Input: part model. Units: mm. Frame: model coordinates. A direction names the side the tool comes from. Coordinates: 2 decimals unless noted, no trailing zeros. Write each loop counter-clockwise with the first axis right and the second up, starting at its lowest first coordinate (ties: lowest second). Pieces come first, ordered by that corner, then holes.
1) Section query D-D (x = -4.5). Output: boundary loops of the cut face in (y, z).
2) Section query C-C (z = 0). Output: boundary loops of the cut face in (x, y), then the cut area to 3 significant figures.
3) Section query B-B (y = 0). Output: boundary loops of the cut face in (x, z).
4) Set-up query: faces 4 (the cylindrical face through (-14.32, -0.95, -0.04)), 5 (the flat face through (-14, 1.85, 0)), 6 (the flat face through (-14, -1.85, 0)), 7 (the flat face through (14, -1.85, 0)). Return all of +Z, -Z, +X, -X, +Y, -Y with unobstructed straight access to the full face (end or side cutting, diameter ignored); none if empty.
5) Section query A-A (x = 14). Output: boundary loops of the cut face in (y, z) (3 decimals).
6) Draft query along Z for faces 1 (the cylindrical face through (14.32, -0.95, 0.04)), 2 (the flat face through (14, 1.85, 0)), 3 (the flat face through (10.35, 0, 0)). Return one class per face: pulls with the +Z half, pulls with the -Z half, needs draft (parallel to the pull), parting line crosses it, or undercut.
7) Line query: L1, parallel to Z at x = -13, y = 0; L2, parallel to Y at x = -13.25, z = 0; L3, parallel to Z at x = -4, y = 0.1. Output: solid intervals per line, ascending.
8) Pin query (flat end, axial travel): pin 1 Ø0.8 at (y, z) = (-2.5, -0.5) entering from -X; pin 2 Ø1.8 at (x, z) = (12.5, 0) entering from +Y; pin 3 Ø3 at (x, z) = (14.5, -0.5) entering from -Y. Return the tip coordinate at first contact, or that it passes through.
from build123d import *

# Parameters (mm, degrees)
SKETCH037_R  = 2.55
PAD031_DEPTH = 10.35
SKETCH038_R  = 0.95
PAD032_DEPTH = 8.05
SKETCH053_R  = 0.95
PAD045_DEPTH = 8.05


with BuildPart() as part:
    # Sketch037 → Pad031 (new body, symmetric)
    with BuildSketch(Plane.YZ):
        Circle(SKETCH037_R)
    extrude(amount=PAD031_DEPTH, both=True)

    # Sketch038 (on Face3 of Pad031) → Pad032 (join)
    with BuildSketch(Plane.YZ.offset(10.35)):
        with BuildLine():
            ThreePointArc((1.85, 1.754993), (0, 2.55), (-1.85, 1.754993))
            Line((-1.85, 1.754993), (-1.85, -1.754993))
            ThreePointArc((-1.85, -1.754993), (0, -2.55), (1.85, -1.754993))
            Line((1.85, 1.754993), (1.85, -1.754993))
        make_face()
        Circle(SKETCH038_R, mode=Mode.SUBTRACT)
    extrude(amount=PAD032_DEPTH)

    # Sketch053 (on Face9 of Pad032) → Pad045 (join)
    with BuildSketch(Plane(origin=(-10.35, 0, 0), x_dir=(0, 1, 0), z_dir=(-1, 0, 0))):
        with BuildLine():
            Line((-1.85, 1.754993), (-1.85, -1.754993))
            ThreePointArc((-1.85, -1.754993), (0, -2.55), (1.85, -1.754993))
            Line((1.85, -1.754993), (1.85, 1.754993))
            ThreePointArc((1.85, 1.754993), (0, 2.55), (-1.85, 1.754993))
        make_face()
        Circle(SKETCH053_R, mode=Mode.SUBTRACT)
    extrude(amount=PAD045_DEPTH)


solid = part.part
Answer:
1. outline: circle Ø5.1 at (0, 0)
2. outline: (-18.4, -1.85) - (-10.35, -1.85) - (-10.35, -2.55) - (10.35, -2.55) - (10.35, -1.85) - (18.4, -1.85) - (18.4, -0.95) - (10.35, -0.95) - (10.35, 0.95) - (18.4, 0.95) - (18.4, 1.85) - (10.35, 1.85) - (10.35, 2.55) - (-10.35, 2.55) - (-10.35, 1.85) - (-18.4, 1.85) - (-18.4, 0.95) - (-10.35, 0.95) - (-10.35, -0.95) - (-18.4, -0.95) - close
2. area: 135 mm2
3. outline: (-18.4, -2.55) - (18.4, -2.55) - (18.4, -0.95) - (10.35, -0.95) - (10.35, 0.95) - (18.4, 0.95) - (18.4, 2.55) - (-18.4, 2.55) - (-18.4, 0.95) - (-10.35, 0.95) - (-10.35, -0.95) - (-18.4, -0.95) - close
4. face 4: -X
4. face 5: +Z, -Z, -X, +Y
4. face 6: +Z, -Z, -X, -Y
4. face 7: +Z, -Z, +X, -Y
5. outline: (-1.85, -1.755) arc R2.55 ccw to (1.85, -1.755) - (1.85, 1.755) arc R2.55 ccw to (-1.85, 1.755) - close; hole circle Ø1.9 at (0, 0)
6. face 1: undercut
6. face 2: needs draft
6. face 3: undercut
7. L1: z = -2.55 to -0.95, 0.95 to 2.55
7. L2: y = -1.85 to -0.95, 0.95 to 1.85
7. L3: z = -2.55 to 2.55
8. pin 1: stops at x = -10.35
8. pin 2: stops at y = 1.85
8. pin 3: stops at y = -1.85
